from build123d import *

# Parameters (mm, degrees)
SKETCH1_W           = 4.8
SKETCH1_H           = 4.8
BOSS_EXTRUDE1_DEPTH = 20
SKETCH2_W           = 5.2
SKETCH2_H           = 5.2
BOSS_EXTRUDE2_DEPTH = 50
SKETCH3_W           = 17
SKETCH3_H           = 27
BOSS_EXTRUDE3_DEPTH = 10
SKETCH4_W           = 13
SKETCH4_H           = 23
CUT_EXTRUDE1_DEPTH  = 8.5
SKETCH5_W           = 11
SKETCH5_H           = 8.5
CUT_EXTRUDE2_DEPTH  = 8.5
SKETCH6_W           = 5
SKETCH6_H           = 5
BOSS_EXTRUDE4_DEPTH = 81.5
SKETCH7_W           = 5
SKETCH7_H           = 5
BOSS_EXTRUDE5_DEPTH = 43.1
BOSS_EXTRUDE6_DEPTH = 5.2
SKETCH13_W          = 5
SKETCH13_H          = 5
BOSS_EXTRUDE7_DEPTH = 10


with BuildPart() as part:
    # Sketch1 → Boss-Extrude1 (new body)
    with BuildSketch(Plane.XY):
        with Locations((2.4, -2.4)):
            Rectangle(SKETCH1_W, SKETCH1_H)
    extrude(amount=BOSS_EXTRUDE1_DEPTH)

    # Sketch2 → Boss-Extrude2 (add)
    with BuildSketch(Plane(origin=(0, 0, 0), x_dir=(-1, 0, 0), z_dir=(0, 0, -1))):
        with Locations((-2.4, -2.4)):
            Rectangle(SKETCH2_W, SKETCH2_H)
    extrude(amount=BOSS_EXTRUDE2_DEPTH)

    # Sketch3 → Boss-Extrude3 (add)
    with BuildSketch(Plane(origin=(0, 0, -50), x_dir=(-1, 0, 0), z_dir=(0, 0, -1))):
        with Locations((-2.4, -2.4)):
            Rectangle(SKETCH3_W, SKETCH3_H)
    extrude(amount=BOSS_EXTRUDE3_DEPTH)

    # Sketch4 → Cut-Extrude1 (cut)
    with BuildSketch(Plane(origin=(0, 0, -60), x_dir=(-1, 0, 0), z_dir=(0, 0, -1))):
        with Locations((-2.4, -2.4)):
            Rectangle(SKETCH4_W, SKETCH4_H)
    extrude(amount=-CUT_EXTRUDE1_DEPTH, mode=Mode.SUBTRACT)

    # Sketch5 → Cut-Extrude2 (cut)
    with BuildSketch(Plane.XZ.offset(15.9)):
        with Locations((2.4, -54.25)):
            Rectangle(SKETCH5_W, SKETCH5_H)
    extrude(amount=-CUT_EXTRUDE2_DEPTH, mode=Mode.SUBTRACT)

    # Sketch6 → Boss-Extrude4 (add)
    with BuildSketch(Plane(origin=(0, 0.2, 0), x_dir=(1, 0, 0), z_dir=(0, 1, 0))):
        with Locations((2.4, 37.5)):
            Rectangle(SKETCH6_W, SKETCH6_H)
    extrude(amount=-BOSS_EXTRUDE4_DEPTH)

    # Sketch7 → Boss-Extrude5 (add)
    with BuildSketch(Plane(origin=(0, 0, -40), x_dir=(-1, 0, 0), z_dir=(0, 0, -1))):
        with Locations((-2.4, -78.8)):
            Rectangle(SKETCH7_W, SKETCH7_H)
    extrude(amount=BOSS_EXTRUDE5_DEPTH)

    # Sketch12 → Boss-Extrude6 (add)
    with BuildSketch(Plane(origin=(5, 0, 0), x_dir=(0, 0, -1), z_dir=(1, 0, 0))):
        Polygon((13.455782968, -5), (35, -40.359932103), (35, -45.359932103), (8.455782968, -5), align=None)
    extrude(amount=-BOSS_EXTRUDE6_DEPTH)

    # Sketch13 → Boss-Extrude7 (add)
    with BuildSketch(Plane.ZY.offset(0.1)):
        with Locations((-80.6, -78.8)):
            Rectangle(SKETCH13_W, SKETCH13_H)
    extrude(amount=BOSS_EXTRUDE7_DEPTH)


solid = part.part
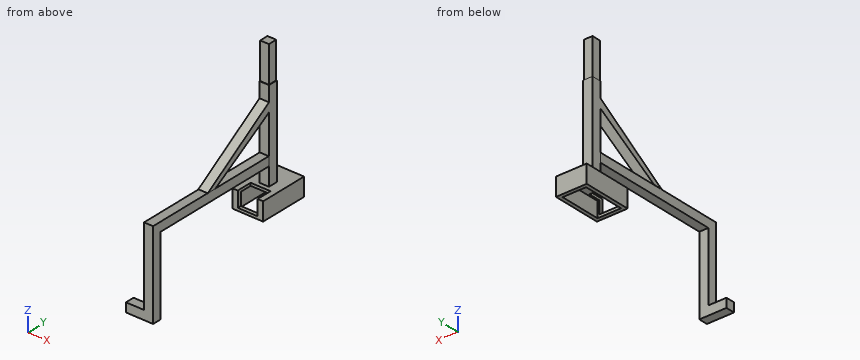
Design review of the part built by this model. Coordinates are the model's own, in mm. Round coordinates to 2 decimals unless told otherwise and drop trailing zeros. Write each loop counter-clockwise with the first axis right and the second up, starting at its lowest first coordinate (ties: lowest second). Pieces come first, ordered by that corner, then holes.
Item 1: Consider section A-A on z = -42.5. Give the boundary of the cut face in (x, y).
Item 2: Consider section D-D on z = -56. Give the boundary of the cut face in (x, y), and give its area (3 significant figures).
Item 3: For pin 1 Ø1 at (y, z) = (0, -1.5) entering from +X; pin 2 Ø8.5 at (x, y) = (2.5, 2) entering from -Z; pin 3 Ø1 at (x, z) = (-0.5, -54.5) entering from -Y; pin 4 Ø10 at (x, y) = (8.5, -5.5) entering from -Z, all flat-tipped, find the tip position at first contact; note any pin that passes through.
Item 4: Consider section B-B on y = -29. Give the boundary of the cut face in (x, z).
Item 5: Wall thickness on L1, parallel to Y at x = 8.5, z = -58.5; L2, parallel to Z at x = 1.5, y = -14.5; L3, parallel to Z at x = 3, y = -61.5: over which ranges is each line inside the solid? List them lowest first.
Item 6: Consider section C-C on y = -11.5. Give the boundary of the cut face in (x, z).
Check values:
1. outline: (-0.2, -5) - (5, -5) - (5, 0.2) - (-0.2, 0.2) - close; (-0.1, -81.3) - (4.9, -81.3) - (4.9, -76.3) - (-0.1, -76.3) - close
2. outline: (-6.1, -15.9) - (-3.1, -15.9) - (-3.1, -13.9) - (-4.1, -13.9) - (-4.1, 9.1) - (8.9, 9.1) - (8.9, -13.9) - (7.9, -13.9) - (7.9, -15.9) - (10.9, -15.9) - (10.9, 11.1) - (-6.1, 11.1) - close; (-0.1, -81.3) - (4.9, -81.3) - (4.9, -76.3) - (-0.1, -76.3) - close
2. area: 163 mm2
3. pin 1: stops at x = 5
3. pin 2: stops at z = -51.5
3. pin 3: stops at y = -81.3
3. pin 4: stops at z = -60
4. outline: (-0.2, -28.08) - (5, -28.08) - (5, -24.24) - (-0.2, -24.24) - close; (-0.1, -40) - (4.9, -40) - (4.9, -35) - (-0.1, -35) - close
5. L1: y = -15.9 to -13.9, 9.1 to 11.1
5. L2: z = -60 to -58.5, -40 to -35, -19.24 to -14.7
5. L3: z = -40 to -35
6. outline: (-6.1, -60) - (-4.1, -60) - (-4.1, -51.5) - (-3.1, -51.5) - (-3.1, -50) - (-6.1, -50) - close; (-0.2, -17.42) - (5, -17.42) - (5, -12.73) - (-0.2, -12.73) - close; (-0.1, -40) - (4.9, -40) - (4.9, -35) - (-0.1, -35) - close; (7.9, -51.5) - (8.9, -51.5) - (8.9, -60) - (10.9, -60) - (10.9, -50) - (7.9, -50) - close
